Read the model definition and answer for the solid it produces. Units are mm, in the model's axes. Give positions to 0.01 mm unless a question says otherwise; leave off trailing zeros. Order: outer loops, then holes, each group sorted by start corner. A loop starts at its lowest first (then second) coordinate and runs counter-clockwise, first axis right, second up.
```python
from build123d import *

# Parameters (mm, degrees)
F0_W        = 12.7
F0_H        = 12.7
F0_R        = 4.8737037562
F1_DEPTH    = 12.7
F3_T1_DEPTH = 50.8


# Not quite as in the source:
# - a fillet or chamfer that OpenCascade refuses, or shapes differently, is made with other operations: its cross-section is extruded or revolved along the edge and cut away or added


with BuildPart() as f1:
    # F0 (on Front) → F1 (new body)
    with BuildSketch(Plane.XZ):
        with Locations((-0.180745963, 2.9901557426)):
            Rectangle(F0_W, F0_H)
        with Locations((0, 2.9901557426)):
            Circle(F0_R, mode=Mode.SUBTRACT)
    extrude(amount=F1_DEPTH)

    # F2: fillet of radius 2.286 on 2 edges, made by hand

    # F2_s1 → F2_t2 (revolve, cut)
    with BuildSketch(Plane.XY.offset(2.9901557426)):
        with BuildLine():
            ThreePointArc((4.8737037562, -10.414), (5.5432576544, -12.0304461018), (7.1597037562, -12.7))
            Line((7.1597037562, -12.7), (4.8737037562, -12.7))
            Line((4.8737037562, -12.7), (4.8737037562, -10.414))
        make_face()
    revolve(axis=Axis((0, -12.7, 2.9901557426), (0, -1, 0)), mode=Mode.SUBTRACT)

    # F2_s3 → F2_t4 (revolve, cut)
    with BuildSketch(Plane.XY.offset(2.9901557426)):
        with BuildLine():
            ThreePointArc((4.8737037562, -2.286), (5.5432576544, -0.6695538982), (7.1597037562, 0))
            Line((7.1597037562, 0), (4.8737037562, 0))
            Line((4.8737037562, 0), (4.8737037562, -2.286))
        make_face()
    revolve(axis=Axis((0, 0, 2.9901557426), (0, -1, 0)), mode=Mode.SUBTRACT)

    # F3: fillet of radius 7.62 on 2 edges, made by hand

    # F3_s2 → F3_t1 (cut)
    with BuildSketch(Plane.XZ.offset(-19.05)):
        with BuildLine():
            ThreePointArc((6.169254037, 4.2601557426), (3.9374077096, -1.12799793), (-1.450745963, -3.3598442574))
            Line((-1.450745963, -3.3598442574), (6.169254037, -3.3598442574))
            Line((6.169254037, -3.3598442574), (6.169254037, 4.2601557426))
        make_face()
        with BuildLine():
            ThreePointArc((-6.530745963, 4.2601557426), (-4.2988996356, -1.12799793), (1.089254037, -3.3598442574))
            Line((1.089254037, -3.3598442574), (-6.530745963, -3.3598442574))
            Line((-6.530745963, -3.3598442574), (-6.530745963, 4.2601557426))
        make_face()
    extrude(amount=F3_T1_DEPTH, mode=Mode.SUBTRACT)


solid = f1.part
```
1) The part is cut by section C-C on y = -11.25. Determine the outline of the cut face in (x, z).
Final values:
outline: (-6.53, 4.26) arc R7.62 ccw to (-0.18, -3.25) arc R7.62 ccw to (6.17, 4.26) - (6.17, 9.34) - (-6.53, 9.34) - close; hole circle Ø10.06 at (0, 2.99)
2) The part is cut by section A-A on x = 0. Determine the outline of the cut face in (y, z), and give its area (3 significant figures).
Final values:
outline: (-12.55, 9.34) arc R2.29 ccw to (-10.41, 7.86) - (-2.29, 7.86) arc R2.29 ccw to (-0.15, 9.34) - close; (-12.49, -3.22) - (-0.21, -3.22) arc R2.29 ccw to (-2.29, -1.88) - (-10.41, -1.88) arc R2.29 ccw to start
area: 31.4 mm2
3) Given pin 1 (5 mm diameter, centred on y = -6.5, z = 1.5, fed in from -X); pin 2 (4 mm diameter, centred on x = -2.5, z = -1, fed in from +Y); pin 3 (6 mm diameter, centred on x = 2.5, y = -8, fed in from -Z), each flat-ended and moving along its own axis, determine where each tip first touches the part or whether it passes through.
Final values:
pin 1: stops at x = -6.53
pin 2: stops at y = -0.28
pin 3: stops at z = -3.25
4) Consider L1, parallel to Z at x = 0.5, y = -0.75; L2, parallel to Z at x = 4.5, y = -3; L3, parallel to X at y = -10.5, z = 3.5. Determine where each line is inside the solid, lowest interval first.
Final values:
L1: z = -3.11 to -2.45, 8.43 to 9.34
L2: z = -0.5 to 1.12, 4.86 to 9.34
L3: x = -6.49 to -4.85, 4.85 to 6.13
5) The part is cut by section B-B on y = -1.5. Determine the outline of the cut face in (x, z).
Final values:
outline: (-6.53, 4.26) arc R7.62 ccw to (-0.18, -3.25) arc R7.62 ccw to (6.17, 4.26) - (6.17, 9.34) - (-6.53, 9.34) - close; hole circle Ø10.03 at (0, 2.99)
6) For a pull along Z with two mould halves and no side action, classify faces 1 (the face through (-6.531, -6, 7)), 2 (the face through (0, -6, 9.34)), 3 (the face through (-0.634, -6.293, 7.822)), 4 (the face through (4.42, -6.26, -0.6)) as released by +Z, released by -Z, zero draft, split by the parting line, or undercut.
Final values:
face 1: zero draft
face 2: released by +Z
face 3: undercut
face 4: released by -Z
